Input: part model. Units: mm. Frame: model coordinates. A direction names the side the tool comes from. Coordinates: 2 decimals unless noted, no trailing zeros. Loops run counter-clockwise (first coordinate to the right, second up) from the corner with the lowest first, then second, coordinate; pieces in that order, holes last. Notation, with made-up numbers: M 13.25,19 L 37.25,19 A30 ccw 37.25,49 Z; hole C 50,-27 d5. An arc over 180 degrees is marked long. Use a Markdown table: item, result. Add a question column.
1. Section A-A on y = -31.75. Output: boundary loops of the cut face in (x, z) (3 decimals), then the cut area to 3 significant figures.
2. Section D-D on x = 5.5. Output: boundary loops of the cut face in (y, z), then the cut area to 3 significant figures.
3. Draft query along X for faces 1 (the flat face through (25.4, -28, 25)), 2 (the cylindrical face through (31.66, -31.06, 15.95)), 3 (the flat face through (38.1, -23, 25)). Return one class per face: +X half, -X half, draft (parallel to the pull), parting line (faces both ways), or undercut.
4. Set-up query: faces 4 (the flat face through (-5.499, -6, 25)), 5 (the flat face through (-1, -12, 0)), 6 (the flat face through (-6, -12.7, 25)). Return all of +Z, -Z, +X, -X, +Y, -Y with unobstructed straight access to the full face (end or side cutting, diameter ignored); none if empty.
5. Line query: L1, parallel to Z at x = 33.5, y = -31.75 (3 decimals); L2, parallel to X at y = -34.5, z = 38.5; L3, parallel to Y at x = -32, z = 19. Output: solid intervals per line, ascending. Write a range as [from, to].
6. Section C-C on y = -40.5. Output: boundary loops of the cut face in (x, z).
7. Pin query (flat end, axial travel): pin 1 (5.5 mm diameter, centred on y = -31.75, z = 19.05, fed in from +X); pin 2 (6 mm diameter, centred on x = 13.5, z = 34, fed in from -Y). Return the tip coordinate at first contact, or that it passes through.
8. Section B-B on z = 9.5. Output: boundary loops of the cut face in (x, y).
```python
from build123d import *

# Parameters (mm, degrees)
BOSS_EXTRUDE1_DEPTH = 50.8
CUT_EXTRUDE1_REACH  = 79.512
SKETCH4_R           = 3.175
CUT_EXTRUDE2_DEPTH  = 83.8


with BuildPart() as part:
    # Sketch2 → Boss-Extrude1 (new body)
    with BuildSketch(Plane.XY):
        Polygon((38.1, 0), (-38.1, 0), (-38.1, -44.45), (-25.4, -44.45), (-25.4, -12.7), (25.4, -12.7), (25.4, -44.45), (38.1, -44.45), align=None)
    extrude(amount=BOSS_EXTRUDE1_DEPTH)

    # Sketch3 → Cut-Extrude1 (cut, up to next)
    with BuildSketch(Plane(origin=(0, 0, 0), x_dir=(1, 0, 0), z_dir=(0, 1, 0)), mode=Mode.PRIVATE) as cut_extrude1_sk1:
        with BuildLine():
            ThreePointArc((6.35, -25.4), (1.643500936, -19.266371003), (-5.499261314, -22.225))
            Line((-5.499261314, -22.225), (-5.499261314, -28.575))
            ThreePointArc((-5.499261314, -28.575), (1.643500936, -31.533628997), (6.35, -25.4))
        make_face()
    cut_extrude1_tool1 = extrude(cut_extrude1_sk1.sketch, amount=-CUT_EXTRUDE1_REACH, mode=Mode.PRIVATE) & part.part
    add(cut_extrude1_tool1.solids().sort_by_distance((0.17344, 0, 25.4))[0], mode=Mode.SUBTRACT)

    # Sketch4 → Cut-Extrude2 (cut)
    with BuildSketch(Plane.ZY.offset(38.1)):
        with Locations(Location((19.05, -31.75, 0), (0, 0, 270))):
            Circle(SKETCH4_R)
        with Locations(Location((31.75, -31.75, 0), (0, 0, 270))):
            Circle(SKETCH4_R)
    extrude(amount=-CUT_EXTRUDE2_DEPTH, mode=Mode.SUBTRACT)


solid = part.part
```
Answers below:
| question | item | result |
|---|---|---|
| 1 | outline | M -38.1,0 L -25.4,0 L -25.4,15.875 L -38.1,15.875 Z; M -38.1,22.225 L -25.4,22.225 L -25.4,28.575 L -38.1,28.575 Z; M -38.1,34.925 L -25.4,34.925 L -25.4,50.8 L -38.1,50.8 Z; M 25.4,0 L 38.1,0 L 38.1,15.875 L 25.4,15.875 Z; M 25.4,22.225 L 38.1,22.225 L 38.1,28.575 L 25.4,28.575 Z; M 25.4,34.925 L 38.1,34.925 L 38.1,50.8 L 25.4,50.8 Z |
| 1 | area | 968 mm² |
| 2 | outline | M -12.7,0 L 0,0 L 0,22.23 L -12.7,22.23 Z; M -12.7,28.57 L 0,28.57 L 0,50.8 L -12.7,50.8 Z |
| 2 | area | 565 mm² |
| 3 | face 1 | undercut |
| 3 | face 2 | draft |
| 3 | face 3 | +X half |
| 4 | face 4 | +Y, -Y |
| 4 | face 5 | -Z, +X, -X, +Y, -Y |
| 4 | face 6 | +Z, -Z, -Y |
| 5 | L1 | z = [0, 15.875], [22.225, 28.575], [34.925, 50.8] |
| 5 | L2 | x = [-38.1, -25.4], [25.4, 38.1] |
| 5 | L3 | y = [-44.45, -34.92], [-28.58, 0] |
| 6 | outline | M -38.1,0 L -25.4,0 L -25.4,50.8 L -38.1,50.8 Z; M 25.4,0 L 38.1,0 L 38.1,50.8 L 25.4,50.8 Z |
| 7 | pin 1 | passes through |
| 7 | pin 2 | stops at y = -12.7 |
| 8 | outline | M -38.1,-44.45 L -25.4,-44.45 L -25.4,-12.7 L 25.4,-12.7 L 25.4,-44.45 L 38.1,-44.45 L 38.1,0 L -38.1,0 Z |
